```python
from build123d import *

# Parameters (mm, degrees)
BOSS_EXTRUDE1_DEPTH = 8
SKETCH2_R           = 16
SKETCH2_R_2         = 11
CUT_EXTRUDE1_DEPTH  = 1
SKETCH3_R           = 3
BOSS_EXTRUDE2_DEPTH = 10
SKETCH4_R           = 2
CUT_EXTRUDE2_DEPTH  = 32.336879232
BOSS_EXTRUDE4_START = 2
SKETCH5_R           = 11
BOSS_EXTRUDE4_DEPTH = 2
SKETCH6_R           = 3
BOSS_EXTRUDE5_DEPTH = 14


with BuildPart() as part:
    # Sketch1 → Boss-Extrude1 (new body)
    with BuildSketch(Plane(origin=(0, 0, 0), x_dir=(1, 0, 0), z_dir=(0, 1, 0))):
        Polygon((-21, 20), (-20, 21), (20, 21), (21, 20), (21, -20), (20, -21), (-20, -21), (-21, -20), align=None)
    extrude(amount=BOSS_EXTRUDE1_DEPTH)

    # Sketch2 → Cut-Extrude1 (cut)
    with BuildSketch(Plane(origin=(0, 8, 0), x_dir=(1, 0, 0), z_dir=(0, 1, 0))):
        with Locations(Location((0, 0, 0), (0, 0, 270))):
            Circle(SKETCH2_R)
        with Locations(Location((0, 0, 0), (0, 0, 270))):
            Circle(SKETCH2_R_2, mode=Mode.SUBTRACT)
    extrude(amount=-CUT_EXTRUDE1_DEPTH, mode=Mode.SUBTRACT)

    # Sketch3 → Boss-Extrude2 (add)
    with BuildSketch(Plane(origin=(0, 8, 0), x_dir=(1, 0, 0), z_dir=(0, 1, 0))):
        with Locations(Location((0, 0, 0), (0, 0, 90))):
            Circle(SKETCH3_R)
    extrude(amount=BOSS_EXTRUDE2_DEPTH)

    # Sketch4 → Cut-Extrude2 (cut, through all)
    with BuildSketch(Plane(origin=(0, 8, 0), x_dir=(1, 0, 0), z_dir=(0, 1, 0))):
        with Locations(Location((-15.5, 15.5, 0), (0, 0, 270))):
            Circle(SKETCH4_R)
        with Locations(Location((15.5, 15.5, 0), (0, 0, 270))):
            Circle(SKETCH4_R)
        with Locations(Location((15.5, -15.5, 0), (0, 0, 270))):
            Circle(SKETCH4_R)
        with Locations(Location((-15.5, -15.5, 0), (0, 0, 270))):
            Circle(SKETCH4_R)
    extrude(amount=-CUT_EXTRUDE2_DEPTH, mode=Mode.SUBTRACT)

    # Sketch5 → Boss-Extrude4 (add)
    with BuildSketch(Plane(origin=(0, 8, 0), x_dir=(1, 0, 0), z_dir=(0, 1, 0)).offset(BOSS_EXTRUDE4_START)):
        with Locations(Location((0, 0, 0), (0, 0, 270))):
            Circle(SKETCH5_R)
    extrude(amount=-BOSS_EXTRUDE4_DEPTH)

    # Sketch6 → Boss-Extrude5 (add)
    with BuildSketch(Plane(origin=(0, 18, 0), x_dir=(1, 0, 0), z_dir=(0, 1, 0))):
        with Locations(Location((0, 0, 0), (0, 0, 270))):
            Circle(SKETCH6_R)
    extrude(amount=BOSS_EXTRUDE5_DEPTH)


solid = part.part
```
Can you work these out from the model? Positions are in its coordinate system, mm. A direction names the side the tool comes from. Coordinates: 2 decimals unless noted, no trailing zeros. Loops run counter-clockwise (first coordinate to the right, second up) from the corner with the lowest first, then second, coordinate; pieces in that order, holes last. Notation, with made-up numbers: (8, 21.5) - (26, 21.5) arc R31 ccw to (26, 50.5) - close; hole circle Ø1 at (-17.5, -31.75). An arc over 180 degrees is marked (long way). Use a Markdown table: item, result.
Item 1: I want a section at C-C on x = 0. Please give me the cut outline in (y, z).
Numbers:
| item | result |
|---|---|
| outline | (0, -21) - (8, -21) - (8, -16) - (7, -16) - (7, -11) - (10, -11) - (10, -3) - (32, -3) - (32, 3) - (10, 3) - (10, 11) - (7, 11) - (7, 16) - (8, 16) - (8, 21) - (0, 21) - close |
Item 2: I want a section at B-B on z = 0. Please give me the cut outline in (x, y), and give its area (3 significant figures).
Numbers:
| item | result |
|---|---|
| outline | (-21, 0) - (21, 0) - (21, 8) - (16, 8) - (16, 7) - (11, 7) - (11, 10) - (3, 10) - (3, 32) - (-3, 32) - (-3, 10) - (-11, 10) - (-11, 7) - (-16, 7) - (-16, 8) - (-21, 8) - close |
| area | 502 mm2 |
Item 3: I want a section at A-A on y = 4.5. Please give me the cut outline in (x, z).
Numbers:
| item | result |
|---|---|
| outline | (-21, -20) - (-20, -21) - (20, -21) - (21, -20) - (21, 20) - (20, 21) - (-20, 21) - (-21, 20) - close; hole circle Ø4 at (-15.5, -15.5); hole circle Ø4 at (-15.5, 15.5); hole circle Ø4 at (15.5, -15.5); hole circle Ø4 at (15.5, 15.5) |
Item 4: I want a section at D-D on y = 12. Please give me the cut outline in (x, z).
Numbers:
| item | result |
|---|---|
| outline | circle Ø6 at (0, 0) |
Item 5: If I drill on probe 1 along X at (y, z) = (5, -15.5); probe 2 along X at (y, z) = (7.5, 0); probe 3 along Z at (x, y) = (15, 4), over which ranges is the centre line in solid material (lowest first)? Write a range as from..to.
Numbers:
| item | result |
|---|---|
| probe 1 | x = -21..-17.5, -13.5..13.5, 17.5..21 |
| probe 2 | x = -21..-16, -11..11, 16..21 |
| probe 3 | z = -21..-17.44, -13.56..13.56, 17.44..21 |
Item 6: Will these pins go through, and if not, where does the flat tip stop? pin 1 (2 mm diameter, centred on x = -1.5, y = 18, fed in from -Z); pin 2 (1 mm diameter, centred on y = 15, z = 2, fed in from +X); pin 3 (12 mm diameter, centred on x = -0.5, y = 21, fed in from +Z); pin 4 (3 mm diameter, centred on x = -15.5, z = -15.5, fed in from -Y).
Numbers:
| item | result |
|---|---|
| pin 1 | stops at z = -2.96 |
| pin 2 | stops at x = 2.6 |
| pin 3 | stops at z = 3 |
| pin 4 | passes through |
Item 7: For faces 4 (the face through (-13.517, 4.056, 15.24)), 5 (the face through (-9, 8, 14)), which set-ups out of +Z, -Z, +X, -X, +Y, -Y let a thin tool reach every point of the face, with its end or its side?
Numbers:
| item | result |
|---|---|
| face 4 | +Y, -Y |
| face 5 | +Y |
Item 8: We'd pull the mould along Z, two halves only. Please class faces 1 (the face through (0, 4, -21)), 2 (the face through (-2.3, 10, 2.3)), 3 (the face through (-15.62, 7.51, -3.47)): released by +Z, released by -Z, zero draft, split by the parting line, or undercut.
Numbers:
| item | result |
|---|---|
| face 1 | released by -Z |
| face 2 | zero draft |
| face 3 | undercut |
